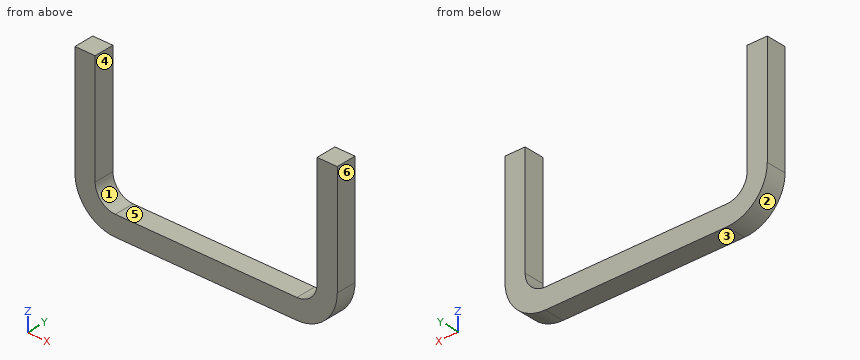
from build123d import *

# Parameters (mm, degrees)
F2_W = 6.35
F2_H = 6.35


with BuildPart() as f3:
    # F3: sweep along a path in F0
    with BuildLine(Plane.XZ) as f3_path:
        Line((-38.1, 44.45), (-38.1, 9.525))
        ThreePointArc((-38.1, 9.525), (-35.3101920908, 2.7898079092), (-28.575, 0))
        Line((-28.575, 0), (0, 0))
        Line((0, 0), (28.575, 0))
        ThreePointArc((28.575, 0), (35.3101920908, 2.7898079092), (38.1, 9.525))
        Line((38.1, 9.525), (38.1, 44.45))
    # F2 (on offset) → F3 (sweep)
    with BuildSketch(Plane.XY.offset(44.45)):
        with Locations((-38.1, 0)):
            Rectangle(F2_W, F2_H)
    sweep(path=f3_path.line)


solid = f3.part
Here's how the part is built. I have some questions about the finished solid (model axes, mm). Face numbers are marked on the shaded views. A direction names the side the tool comes from. Round coordinates to 2 decimals unless told otherwise and drop trailing zeros. Write each loop counter-clockwise with the first axis right and the second up, starting at its lowest first coordinate (ties: lowest second). Pieces come first, ordered by that corner, then holes. Notation, with made-up numbers: (86.25, -5.75) -> (115.25, -5.75) arc R25 cw to (115.25, 6.25) -> close; hole circle Ø11 at (-21.75, 80.25). An arc over 180 degrees is marked (long way). One line per item, written item: value.
1) Suppose I cut it at B-B on y = -2.25. List the corners of the cut face in (x, z) for me (3 decimals).
Filled sheet:
outline: (-41.275, 9.525) arc R12.7 ccw to (-28.575, -3.175) -> (28.575, -3.175) arc R12.7 ccw to (41.275, 9.525) -> (41.275, 44.45) -> (34.925, 44.45) -> (34.925, 9.525) arc R6.35 cw to (28.575, 3.175) -> (-28.575, 3.175) arc R6.35 cw to (-34.925, 9.525) -> (-34.925, 44.45) -> (-41.275, 44.45) -> close
2) I'm going to push flat-ended pins straight in: pin 1 Ø2 at (x, y) = (12, -1) entering from +Z (3 decimals); pin 2 Ø2 at (y, z) = (2, 2.5) entering from -X. Where does each tip first touch, or does it pass through?
Filled sheet:
pin 1: stops at z = 3.175
pin 2: stops at x = -39.75
3) If I drill on line 1 (X direction, y = 0.75, z = 13) (3 decimals); line 2 (Z direction, x = -24, y = -1) (3 decimals); line 3 (X direction, y = -0.75, z = 8), over which ranges is the centre line in solid material (lowest first)? Write a range as [from, to].
Filled sheet:
line 1: x = [-41.275, -34.925], [34.925, 41.275]
line 2: z = [-3.175, 3.175]
line 3: x = [-41.18, -34.74], [34.74, 41.18]
4) For the marked faces 5 and 6, which set-ups out of +Z, -Z, +X, -X, +Y, -Y let a thin tool reach every point of the face, with its end or its side?
Filled sheet:
face 5: +Z, +Y, -Y
face 6: +Z, -Z, +X, +Y, -Y
5) Suppose I cut it at C-C on x = 6. List the corners of the cut face in (y, z) for me (3 decimals).
Filled sheet:
outline: (-3.175, -3.175) -> (3.175, -3.175) -> (3.175, 3.175) -> (-3.175, 3.175) -> close
6) Suppose I cut it at A-A on z = 41. List the corners of the cut face in (x, y) for me (3 decimals), plus the area to 3 significant figures.
Filled sheet:
outline: (-41.275, -3.175) -> (-34.925, -3.175) -> (-34.925, 3.175) -> (-41.275, 3.175) -> close; (34.925, -3.175) -> (41.275, -3.175) -> (41.275, 3.175) -> (34.925, 3.175) -> close
area: 80.6 mm2
7) We'd pull the mould along X, two halves only. Please class the marked faces 1, 2, 3 and 4: released by +X, released by -X, zero draft, split by the parting line, or undercut.
Filled sheet:
face 1: undercut
face 2: released by -X
face 3: zero draft
face 4: undercut
